from build123d import *

# Parameters (mm, degrees)
F0_W     = 60
F0_H     = 20
F1_DEPTH = 20
F2_W     = 10
F2_H     = 20
F3_DEPTH = 10
F4_W     = 10
F4_H     = 10
F5_DEPTH = 20
F6_R     = 4.99999


# Not quite as in the source:
# - a fillet or chamfer is up to 0.001 mm smaller than in the source, because OpenCascade refuses the exact size


with BuildPart() as f1:
    # F0 (on Top) → F1 (new body)
    with BuildSketch(Plane.XY):
        with Locations((30, -10)):
            Rectangle(F0_W, F0_H)
    extrude(amount=F1_DEPTH)

    # F2 (on face) → F3 (cut)
    with BuildSketch(Plane.XY.offset(20)):
        with Locations((25, -10)):
            Rectangle(F2_W, F2_H)
    extrude(amount=-F3_DEPTH, mode=Mode.SUBTRACT)

    # F4 (on face) → F5 (cut)
    with BuildSketch(Plane.XY.offset(20)):
        with Locations((35, -5)):
            Rectangle(F4_W, F4_H)
    extrude(amount=-F5_DEPTH, mode=Mode.SUBTRACT)

    # F6 (radius 5 in the source; OpenCascade refuses exactly that, so slightly less here)
    f6_edges = [f1.edges().sort_by_distance(p)[0] for p in [
        (30, -10, 5),
        (40, -10, 10),
    ]]
    fillet(f6_edges, radius=F6_R)


solid = f1.part
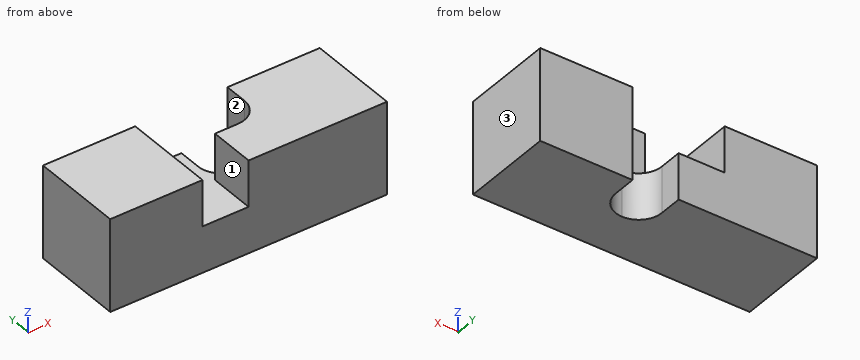
Can you work these out from the model? Positions are in its coordinate system, mm. Face numbers are marked on the shaded views. A direction names the side the tool comes from. Round coordinates to 2 decimals unless told otherwise and drop trailing zeros. Loops run counter-clockwise (first coordinate to the right, second up) from the corner with the lowest first, then second, coordinate; pieces in that order, holes last. Notation, with made-up numbers: (9.5, -25) - (42.5, -25) arc R26 cw to (42.5, 10) - close; hole circle Ø4 at (22, -30). An arc over 180 degrees is marked (long way). Write item = value, one per line. Start each with the question number.
(1) If I drill on probe 1 along X at (y, z) = (-2.5, 11.5); probe 2 along X at (y, z) = (-4.25, 7); probe 3 along Z at (x, y) = (23, -3.5), over which ranges is the centre line in solid material (lowest first)? Write a range as [from, to].
(2) If we section it at D-D (y = -15.5): Please give me the cut outline in (x, z).
(3) For P1, Ø1.5, axis at x = 32.5, z = 9, coming from the +Y side, with a flat end and sliding along its axis, tell me the tip position at first contact or that it passes through.
(4) If we section it at A-A (y = -9): Please give me the cut outline in (x, z), and give its area (3 significant figures).
(5) If we section it at B-B (z = 11): Please give me the cut outline in (x, y).
(6) For the marked faces 1, 2 and 3, which set-ups out of +Z, -Z, +X, -X, +Y, -Y let a thin tool reach every point of the face, with its end or its side?
Ans:
q1.probe_1 = [0, 20], [40, 60]
q1.probe_2 = [0, 30], [40, 60]
q1.probe_3 = [0, 10]
q2.outline = (0, 0) - (60, 0) - (60, 20) - (30, 20) - (30, 10) - (20, 10) - (20, 20) - (0, 20) - close
q3.P1 = -8.8
q4.outline = (0, 0) - (32, 0) - (32, 10) - (20, 10) - (20, 20) - (0, 20) - close; (38, 0) - (60, 0) - (60, 20) - (38, 20) - close
q4.area = 960 mm²
q5.outline = (0, -20) - (20, -20) - (20, 0) - (0, 0) - close; (30, -20) - (60, -20) - (60, 0) - (40, 0) - (40, -5) arc R5 cw to (35, -10) - (30, -10) - close
q6.face_1 = +Z, +Y, -Y
q6.face_2 = +Z, -Z, +Y
q6.face_3 = +Z, -Z, +X, +Y, -Y
